For this review, use the dimensioned drawing (mm, ordinates from the lowest corner) and the shaded views. A direction names the side the tool comes from. Give positions to 0.01 mm unless a question says otherwise; leave off trailing zeros. Loops run counter-clockwise (first coordinate to the right, second up) from the corner with the lowest first, then second, coordinate; pieces in that order, holes last. Notation, with made-up numbers: (-23, 52) - (14, 52) arc R23 ccw to (14, 88) - close; hole circle Ø8 at (43, 20). An arc over 180 degrees is marked (long way). Put each result on its own line as item: value.
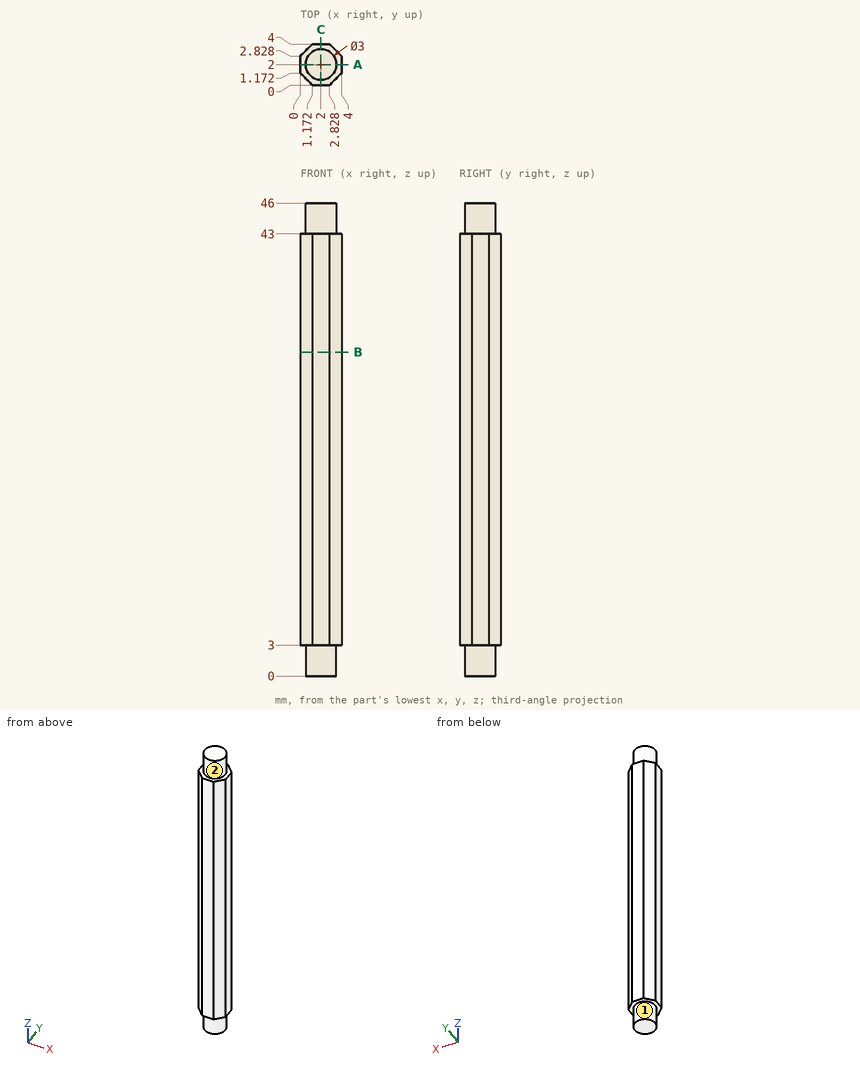
1) For the marked faces 1 and 2, list the 3-axis set-ups (+Z, -Z, +X, -X, +Y, -Y) from which the entire face can be reached by the end or side of a thin tool; tool diameter is ignored.
Geometry check:
face 1: -Z
face 2: +Z
2) Take a section at B-B on z = 31.5. State the section outline as (x, y) points.
Geometry check:
outline: (0, 1.17) - (1.17, 0) - (2.83, 0) - (4, 1.17) - (4, 2.83) - (2.83, 4) - (1.17, 4) - (0, 2.83) - close
3) Take a section at A-A on y = 2. State the section outline as (x, z) points, and give its area (3 significant figures).
Geometry check:
outline: (0, 3) - (0.5, 3) - (0.5, 0) - (3.5, 0) - (3.5, 3) - (4, 3) - (4, 43) - (3.5, 43) - (3.5, 46) - (0.5, 46) - (0.5, 43) - (0, 43) - close
area: 178 mm²
4) Wall thickness on line 1 (Z direction, x = 2.7, y = 3.85); line 2 (X direction, y = 0.9, z = 4); line 3 (Y direction, x = 3.6, z = 13.5): over which ranges is each line inside the solid? List them lowest first.
Geometry check:
line 1: z = 3 to 43
line 2: x = 0.27 to 3.73
line 3: y = 0.77 to 3.23
